from build123d import *

# Parameters (mm, degrees)
SKETCH2_R           = 14.2875
SKETCH2_R_2         = 6.35
SKETCH2_R_3         = 4.064
BOSS_EXTRUDE1_DEPTH = 6.35


with BuildPart() as part:
    # Sketch2 → Boss-Extrude1 (new body)
    with BuildSketch(Plane(origin=(0, 0, 0), x_dir=(1, 0, 0), z_dir=(0, 1, 0))):
        with BuildLine():
            Line((31.75, 20.031971953), (31.75, 117.475))
            ThreePointArc((31.75, 117.475), (27.49630657, 133.35), (15.875, 144.97130657))
            add(Edge.make_bspline(
                [(-11.426385325, 153.835795689), (1.224450482, 152.855976047), (15.875, 144.97130657)],
                knots=[0, 0, 0, 1, 1, 1], degree=2))
            add(Edge.make_bspline(
                [(-64.783506655, 184.207168681), (-52.423507121, 162.771572898), (-33.18367174, 151.627706727), (-11.426385325, 153.835795689)],
                knots=[0, 0, 0, 0, 1, 1, 1, 1], degree=3))
            add(Edge.make_bspline(
                [(-85.86133431, 203.70880657), (-72.386286962, 196.104383794), (-64.783506655, 184.207168681)],
                knots=[0, 0, 0, 1, 1, 1], degree=2))
            ThreePointArc((-85.86133431, 203.70880657), (-129.23264088, 192.0875), (-117.61133431, 148.71619343))
            Line((-117.61133431, 148.71619343), (-57.15, 113.808825791))
            ThreePointArc((-57.15, 113.808825791), (-38.555909488, 95.214735278), (-31.75, 69.814735278))
            Line((-31.75, 69.814735278), (-31.75, -41.275))
            ThreePointArc((-31.75, -41.275), (0, -73.025), (31.75, -41.275))
            Line((31.75, -41.275), (31.75, 20.031971953))
        make_face()
        with Locations(Location((0, 0, 0), (0, 0, 270))):
            Circle(SKETCH2_R, mode=Mode.SUBTRACT)
        with Locations(Location((0, 117.475, 0), (0, 0, 270))):
            Circle(SKETCH2_R, mode=Mode.SUBTRACT)
        with Locations(Location((-101.73633431, 176.2125, 0), (0, 0, 270))):
            Circle(SKETCH2_R, mode=Mode.SUBTRACT)
        with Locations(Location((0, -57.15, 0), (0, 0, 270))):
            Circle(SKETCH2_R_2, mode=Mode.SUBTRACT)
        with Locations(Location((-54.043167155, 141.344488686, 0), (0, 0, 270))):
            Circle(SKETCH2_R_3, mode=Mode.SUBTRACT)
    extrude(amount=BOSS_EXTRUDE1_DEPTH)


solid = part.part
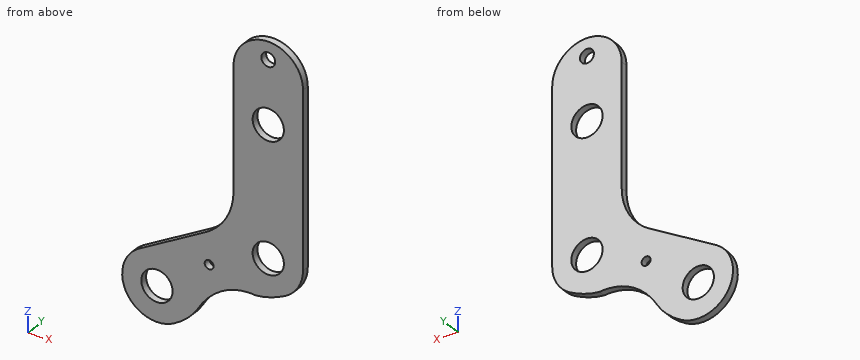
Geometry check sheet. Reference: the model listing, model coordinates, mm. Coordinates: 2 decimals unless noted, no trailing zeros. Order: outer loops, then holes, each group sorted by start corner. A loop starts at its lowest first (then second) coordinate and runs counter-clockwise, first axis right, second up. Notation, with made-up numbers: M 12,-33 L 49,-33 A15 ccw 49,-21 Z; hole C 54,-26.75 d7. An arc over 180 degrees is marked long. Use CSV: the item, a comma, the result in double quotes.
Item 1: Cross-section at C-C on y = 3.75. Give the number of separate pieces and of enclosed holes in the cut face, then the cut area to 3 significant figures.
Returned:
separate pieces,"1"
enclosed holes,"5"
area,"17,800 mm2"
Item 2: Gauge pin test, flat ends, axial feed: pin 1 Ø9.5 at (x, z) = (-54.04, -141.34) entering from +Y; pin 2 Ø3 at (x, y) = (7, 4.5) entering from -Z; pin 3 Ø7.5 at (x, z) = (0, 57.15) entering from +Y. Record the tip position at first contact, or that the pin passes through.
Returned:
pin 1,"stops at y = 6.35"
pin 2,"stops at z = -149.79"
pin 3,"passes through"
Item 3: Cross-section at B-B on z = 57.15. Record the cut outline in (x, y), then the cut area to 3 significant figures.
Returned:
outline,"M -27.5,0 L -6.35,0 L -6.35,6.35 L -27.5,6.35 Z; M 6.35,0 L 27.5,0 L 27.5,6.35 L 6.35,6.35 Z"
area,"269 mm2"
Item 4: Cross-section at A-A on z = 0. Record the cut outline in (x, y).
Returned:
outline,"M -31.75,0 L -14.29,0 L -14.29,6.35 L -31.75,6.35 Z; M 14.29,0 L 31.75,0 L 31.75,6.35 L 14.29,6.35 Z"
Item 5: Thickness scan on line 1 along Z through (x, y) = (-103, 3.25); line 2 along X through (y, z) = (1.5, 0); line 3 along X through (y, z) = (2, -10). Record the ranges inside material, lowest first.
Returned:
line 1,"z = -207.94 to -190.44, -161.98 to -140.28"
line 2,"x = -31.75 to -14.29, 14.29 to 31.75"
line 3,"x = -31.75 to -10.2, 10.2 to 31.75"
